Work out the finished part from the listing and answer in its coordinate system (mm). A direction names the side the tool comes from. Coordinates: 2 decimals unless noted, no trailing zeros. Order: outer loops, then holes, each group sorted by start corner. A loop starts at its lowest first (then second) coordinate and runs counter-clockwise, first axis right, second up. Notation, with made-up numbers: (-26.5, 41.25) -> (-5.5, 41.25) arc R19 cw to (-5.5, 58.25) -> close; hole circle Ø5 at (88, 65.25). An arc over 180 degrees is marked (long way). Use one line per item in the form item = value.
from build123d import *

# Parameters (mm, degrees)
F0_R     = 20.955
F0_R_2   = 19.685
F1_DEPTH = 3.175
F2_DEPTH = 6.35
F3_R     = 6.35


with BuildPart() as f1:
    # F0 (on Top) → F1 (new body)
    with BuildSketch(Plane.XY):
        Circle(F0_R)
        Circle(F0_R_2, mode=Mode.SUBTRACT)
    extrude(amount=F1_DEPTH)

    # F0 (on Top) → F2 (join)
    with BuildSketch(Plane.XY):
        with BuildLine():
            ThreePointArc((23.9050999455, -6.4692674698), (24.5490837421, -3.2630832697), (24.765, 0))
            ThreePointArc((24.765, 0), (19.6285885254, 15.1004548773), (6.35, 23.9370575677))
            ThreePointArc((6.35, 23.9370575677), (4.0651088886, 24.4290833787), (1.7440091422, 24.703515076))
            ThreePointArc((1.7440091422, 24.703515076), (1.8643178935, 24.3286489263), (1.905, 23.9370575677))
            ThreePointArc((1.905, 23.9370575677), (-0.3915913586, 22.0727396742), (-1.7440091422, 24.703515076))
            ThreePointArc((-1.7440091422, 24.703515076), (-4.0651088886, 24.4290833787), (-6.35, 23.9370575677))
            ThreePointArc((-6.35, 23.9370575677), (-21.4471191247, 12.3825), (-23.9050999455, -6.4692674698))
            ThreePointArc((-23.9050999455, -6.4692674698), (-23.1887612414, -8.6940541227), (-22.2658761897, -10.8414013165))
            ThreePointArc((-22.2658761897, -10.8414013165), (-20.1370690632, -10.1581864481), (-18.8250999455, -11.9685287839))
            ThreePointArc((-18.8250999455, -11.9685287839), (-19.3113489683, -13.239815795), (-20.5218670475, -13.8621137596))
            ThreePointArc((-20.5218670475, -13.8621137596), (-19.1236523528, -15.735029256), (-17.5550999455, -17.4677900979))
            ThreePointArc((-17.5550999455, -17.4677900979), (0, -24.765), (17.5550999455, -17.4677900979))
            ThreePointArc((17.5550999455, -17.4677900979), (19.1236523528, -15.735029256), (20.5218670475, -13.8621137596))
            ThreePointArc((20.5218670475, -13.8621137596), (19.0803215513, -11.0160287839), (22.2658761897, -10.8414013165))
            ThreePointArc((22.2658761897, -10.8414013165), (23.1887612414, -8.6940541227), (23.9050999455, -6.4692674698))
        make_face()
        Circle(F0_R, mode=Mode.SUBTRACT)
        with BuildLine():
            ThreePointArc((1.7440091422, 24.703515076), (4.0651088886, 24.4290833787), (6.35, 23.9370575677))
            ThreePointArc((6.35, 23.9370575677), (0, 30.2870575677), (-6.35, 23.9370575677))
            ThreePointArc((-6.35, 23.9370575677), (-4.0651088886, 24.4290833787), (-1.7440091422, 24.703515076))
            ThreePointArc((-1.7440091422, 24.703515076), (0, 25.8420575677), (1.7440091422, 24.703515076))
        make_face()
        with BuildLine():
            ThreePointArc((17.5550999455, -17.4677900979), (26.2293612595, -15.1435287839), (23.9050999455, -6.4692674698))
            ThreePointArc((23.9050999455, -6.4692674698), (23.1887612414, -8.6940541227), (22.2658761897, -10.8414013165))
            ThreePointArc((22.2658761897, -10.8414013165), (22.5404422812, -11.3754979015), (22.6350999455, -11.9685287839))
            ThreePointArc((22.6350999455, -11.9685287839), (22.0013869566, -13.3872797611), (20.5218670475, -13.8621137596))
            ThreePointArc((20.5218670475, -13.8621137596), (19.1236523528, -15.735029256), (17.5550999455, -17.4677900979))
        make_face()
        with BuildLine():
            ThreePointArc((-22.2658761897, -10.8414013165), (-23.1887612414, -8.6940541227), (-23.9050999455, -6.4692674698))
            ThreePointArc((-23.9050999455, -6.4692674698), (-26.2293612595, -15.1435287839), (-17.5550999455, -17.4677900979))
            ThreePointArc((-17.5550999455, -17.4677900979), (-19.1236523528, -15.735029256), (-20.5218670475, -13.8621137596))
            ThreePointArc((-20.5218670475, -13.8621137596), (-22.3798783397, -12.9210287839), (-22.2658761897, -10.8414013165))
        make_face()
    extrude(amount=F2_DEPTH)

    # F3
    f3_edges = [f1.edges().sort_by_distance(p)[0] for p in [
        (6.35, 23.937058, 3.175),
        (-23.9051, -6.469267, 3.175),
        (17.5551, -17.46779, 3.175),
        (23.9051, -6.469267, 3.175),
        (-6.35, 23.937058, 3.175),
        (-17.5551, -17.46779, 3.175),
    ]]
    fillet(f3_edges, radius=F3_R)


solid = f1.part
(1) Section A-A on x = 0 is taken. Write down the section's boundary in (y, z) (3 decimals).
Data:
outline = (-24.765, 0) -> (-19.685, 0) -> (-19.685, 3.175) -> (-20.955, 3.175) -> (-20.955, 6.35) -> (-24.765, 6.35) -> close; (19.685, 0) -> (22.032, 0) -> (22.032, 6.35) -> (20.955, 6.35) -> (20.955, 3.175) -> (19.685, 3.175) -> close; (25.842, 0) -> (30.287, 0) -> (30.287, 6.35) -> (25.842, 6.35) -> close
(2) Section D-D on z = 5.5 is taken. Count the separate pieces of the cut face and the enclosed holes in it, plus the area to 3 significant figures.
Data:
separate_pieces = 1
enclosed_holes = 4
area = 691 mm²
(3) Straight lines are drawn through the part: line 1 along Z through (x, y) = (14, -14.5) (3 decimals); line 2 along Y through (x, z) = (-4.5, 0.5); line 3 along X through (y, z) = (17, 3). For each, find the intervals that lie inside material, in ascending order.
Data:
line_1 = 0 to 3.175
line_2 = -24.35 to -19.16, 19.16 to 28.42
line_3 = -18.01 to -9.92, 9.92 to 18.01
(4) Section C-C on y = -16 is taken. Write down the section's boundary in (x, z) (3 decimals), plus the area to 3 significant figures.
Data:
outline = (-25.636, 0) -> (-11.467, 0) -> (-11.467, 3.175) -> (-13.532, 3.175) -> (-13.532, 6.35) -> (-25.636, 6.35) -> close; (11.467, 0) -> (25.636, 0) -> (25.636, 6.35) -> (13.532, 6.35) -> (13.532, 3.175) -> (11.467, 3.175) -> close
area = 167 mm²
(5) Which of the six approach directions +Z, -Z, +X, -X, +Y, -Y give full straight-line access (tool end or side, diameter ignored) to faces 5 (the cylindrical face through (-2.728, 20.777, 4.74)), 6 (the flat face through (-0.1, 21.2, 6.35))?
Data:
face_5 = +Z
face_6 = +Z, +X, -X, +Y, -Y
(6) Each of these flat-tipped pins is pushed along its axis until it touches: P1, Ø1.5, axis at x = 7.5, z = 4.5, coming from the -Y side; P2, Ø3, axis at x = 21.5, z = 5, coming from the -Y side; P3, Ø2.5, axis at x = 20.73, y = -11.97, coming from the -Z side; P4, Ø2, axis at x = -16.5, z = 5, coming from the +Y side. Where does it stop, or does it pass through?
Data:
P1 = -23.83
P2 = -18.32
P3 = through
P4 = 19.31
(7) The mould has two halves that part along Y. Classify faces 1 (the flat face through (-10.2, 17.2, 0)), 2 (the cylindrical face through (-26.281, -15.053, 3.131)), 3 (the flat face through (-19, -6, 3.175)), 4 (the cylindrical face through (-15.62, -11.98, 1.57)): released by +Y, released by -Y, zero draft, split by the parting line, or undercut.
Data:
face_1 = zero draft
face_2 = split by the parting line
face_3 = undercut
face_4 = undercut
(8) Section B-B on y = 18.5 is taken. Write down the section's boundary in (x, z) (3 decimals).
Data:
outline = (-16.464, 0) -> (-6.727, 0) -> (-6.727, 3.175) -> (-9.842, 3.175) -> (-9.842, 6.35) -> (-16.464, 6.35) -> close; (6.727, 0) -> (16.464, 0) -> (16.464, 6.35) -> (9.842, 6.35) -> (9.842, 3.175) -> (6.727, 3.175) -> close
